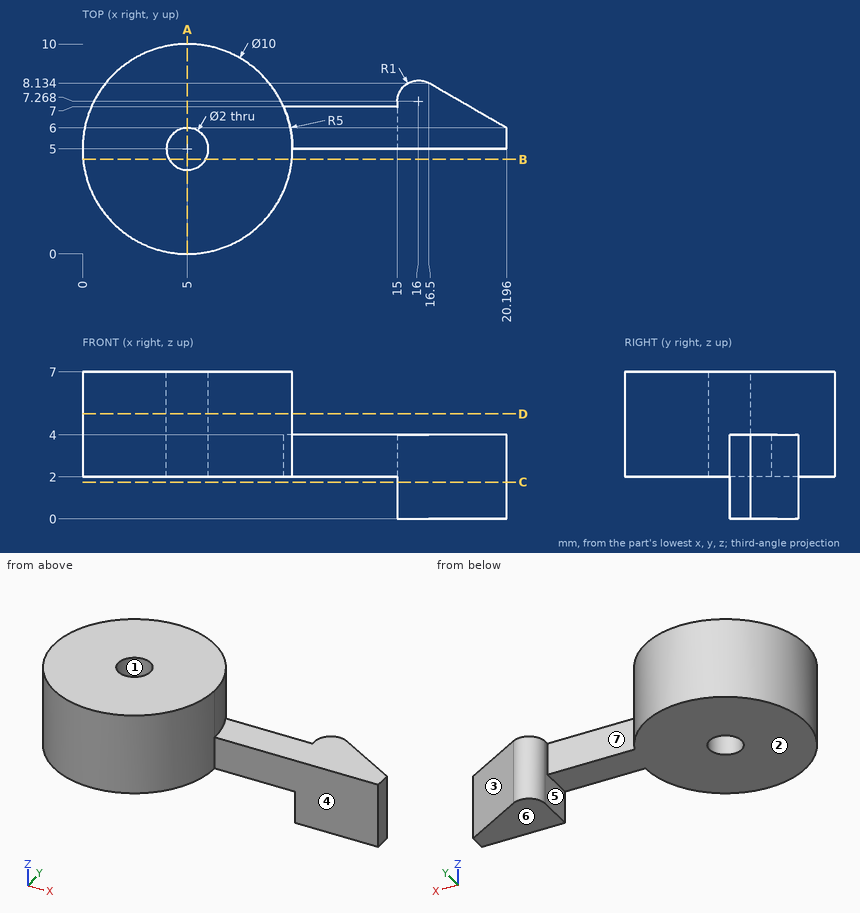
Study the drawing (mm; zero at the part's minimum x, y, z) and answer. A direction names the side the tool comes from. Coordinates: 2 decimals unless noted, no trailing zeros. Loops run counter-clockwise (first coordinate to the right, second up) from the corner with the lowest first, then second, coordinate; pieces in that order, holes last. Notation, with made-up numbers: M -9.5,-36.75 L 36.5,-36.75 A5 cw 36.5,-27.75 Z; hole C -1.75,14 d6. An arc over 180 degrees is marked long. Answer as a JSON object with one key per item and string values. Group by question number.
Item 1: Section D-D (z = 5) is taken. Write down the section's boundary in (x, y), and give its area (3 significant figures).
Item 2: Section B-B (y = 4.5) is taken. Write down the section's boundary in (x, z) (3 decimals).
Item 3: Each of these flat-tipped pins is pushed along its axis until it touches: P1, Ø0.6, axis at x = 12, z = 3, coming from the +Y side; P2, Ø1.5, axis at x = 8, z = 1.5, coming from the +Y side; P3, Ø1.1, axis at y = 6, z = 2, coming from the -X side. Where does it stop, or does it pass through?
Item 4: Which of the six approach directions +Z, -Z, +X, -X, +Y, -Y give full straight-line access (tool end or side, diameter ignored) to the marked faces 4, 5, 6 and 7?
Item 5: Section A-A (x = 5) is taken. Write down the section's boundary in (y, z).
Item 6: Determine the mould class of the marked faces 1, 2 and 3 for opening direction X: +X half, -X half, draft (parallel to the pull), parting line (faces both ways), or undercut.
Item 7: Section C-C (z = 1.75) is taken. Write down the section's boundary in (x, y), and give its area (3 significant figures).
Item 8: Consider L1, parallel to Y at x = 5, z = 4.3; L2, parallel to Y at x = 13, z = 2.25; L3, parallel to Z at x = 3.5, y = 5.5. Determine where each line is inside the solid, lowest interval first.
Solved:
{
 "1": {"outline": "C 5,5 d10; hole C 5,5 d2", "area": "75.4 mm2"},
 "2": {"outline": "M 0.025,2 L 4.134,2 L 4.134,7 L 0.025,7 Z; M 5.866,2 L 9.975,2 L 9.975,7 L 5.866,7 Z"},
 "3": {"P1": "stops at y = 7", "P2": "stops at y = 9.36", "P3": "stops at x = 0.02"},
 "4": {"face 4": "+Z, -Z, +X, -Y", "face 5": "-Z, +Y", "face 6": "-Z, +X, -X, +Y, -Y", "face 7": "+Z, -Z, +Y"},
 "5": {"outline": "M 0,2 L 4,2 L 4,7 L 0,7 Z; M 6,2 L 10,2 L 10,7 L 6,7 Z"},
 "6": {"face 1": "undercut", "face 2": "draft", "face 3": "+X half"},
 "7": {"outline": "M 15,5 L 20.2,5 L 20.2,6 L 16.5,8.13 A1 ccw 15,7.27 Z", "area": "12.3 mm2"},
 "8": {"L1": "y = 0 to 4, 6 to 10", "L2": "y = 5 to 7", "L3": "z = 2 to 7"}
}
